For this review, take the finished solid that the model builds, in its own axes (mm). Face numbers are marked on the shaded views. A direction names the side the tool comes from. Round coordinates to 2 decimals unless told otherwise and drop trailing zeros. Order: outer loops, then holes, each group sorted by start corner. A loop starts at its lowest first (then second) coordinate and runs counter-clockwise, first axis right, second up. Notation, with made-up numbers: (-37.5, -34) -> (-21.5, -34) arc R24 cw to (-21.5, 3) -> close; hole circle Ø8 at (-11, 61.25). An arc over 180 degrees is marked (long way). Use a Markdown table: item, result. Add a question column.
1) Consider section C-C (x = 23.5). State the section outline as (y, z) points.
2) Consider section B-B (y = 27). State the section outline as (x, z) points.
3) Consider section A-A (z = 44). State the section outline as (x, y) points, plus the area to 3 significant figures.
4) Consider section D-D (z = 64.5). State the section outline as (x, y) points.
5) Draft analysis for pull direction Z (two halves, no side actions). For the marked faces 1, 2, 3 and 4, state which applies: pulls with the +Z half, pulls with the -Z half, needs draft (parallel to the pull), parting line crosses it, or undercut.
6) Wall thickness on line 1 along Y through (x, z) = (27, 21); line 2 along X through (y, z) = (3.5, 58); line 3 along Y through (x, z) = (91.5, 16): over which ranges is each line inside the solid? List them lowest first. Write a range as [from, to].
7) Clearance check with flat-ended pins moving along their axes: P1, Ø6, axis at x = 12.5, z = 14.5, coming from the +Y side; P2, Ø10, axis at x = 87.5, y = 42, coming from the +Z side; P3, Ø10, axis at y = 23.5, z = 76.5, coming from the +X side; P4, Ø1, axis at x = 19.5, y = 14.5, coming from the +Z side. State where each tip first meets the part, or that it passes through.
8) Machinability: for the marked faces 5, 6 and 7, which of the approach directions +Z, -Z, +X, -X, +Y, -Y give a long, thin tool a straight path to every point of the face, cutting with its end or side? Answer none if there is none.
```python
from build123d import *

# Parameters (mm, degrees)
SKETCH1_W           = 100
SKETCH1_H           = 30
BOSS_EXTRUDE1_DEPTH = 110
SKETCH2_W           = 90
SKETCH2_H           = 10
CUT_EXTRUDE1_DEPTH  = 110
BOSS_EXTRUDE2_DEPTH = 20
CUT_EXTRUDE2_DEPTH  = 20
SKETCH5_W           = 50
SKETCH5_H           = 50
CUT_EXTRUDE3_DEPTH  = 20
CUT_EXTRUDE4_DEPTH  = 20


with BuildPart() as part:
    # Sketch1 → Boss-Extrude1 (new body)
    with BuildSketch(Plane.XY):
        with Locations((50, 15)):
            Rectangle(SKETCH1_W, SKETCH1_H)
    extrude(amount=BOSS_EXTRUDE1_DEPTH)

    # Sketch2 → Cut-Extrude1 (cut)
    with BuildSketch(Plane.ZY):
        with Locations((65, 25)):
            Rectangle(SKETCH2_W, SKETCH2_H)
    extrude(amount=-CUT_EXTRUDE1_DEPTH, mode=Mode.SUBTRACT)

    # Sketch3 → Boss-Extrude2 (add)
    with BuildSketch(Plane.XY.offset(20)):
        with BuildLine():
            Line((20, 30), (80, 30))
            ThreePointArc((80, 30), (50, 60), (20, 30))
        make_face()
    extrude(amount=-BOSS_EXTRUDE2_DEPTH)

    # Sketch4 → Cut-Extrude2 (cut)
    with BuildSketch(Plane(origin=(0, 20, 0), x_dir=(1, 0, 0), z_dir=(0, 1, 0))):
        with BuildLine():
            Line((50, -110), (100, -110))
            Line((100, -110), (100, -60))
            ThreePointArc((100, -60), (85.355339059, -95.355339059), (50, -110))
        make_face()
    extrude(amount=-CUT_EXTRUDE2_DEPTH, mode=Mode.SUBTRACT)

    # Sketch5 → Cut-Extrude3 (cut)
    with BuildSketch(Plane(origin=(0, 20, 0), x_dir=(1, 0, 0), z_dir=(0, 1, 0))):
        with Locations((25, -85)):
            Rectangle(SKETCH5_W, SKETCH5_H)
    extrude(amount=-CUT_EXTRUDE3_DEPTH, mode=Mode.SUBTRACT)

    # Sketch6 → Cut-Extrude4 (cut)
    with BuildSketch(Plane(origin=(0, 20, 0), x_dir=(1, 0, 0), z_dir=(0, 1, 0))):
        with BuildLine():
            Line((20, -60), (50, -60))
            Line((50, -60), (50, -90))
            ThreePointArc((50, -90), (71.213203436, -38.786796564), (20, -60))
        make_face()
    extrude(amount=-CUT_EXTRUDE4_DEPTH, mode=Mode.SUBTRACT)


solid = part.part
```
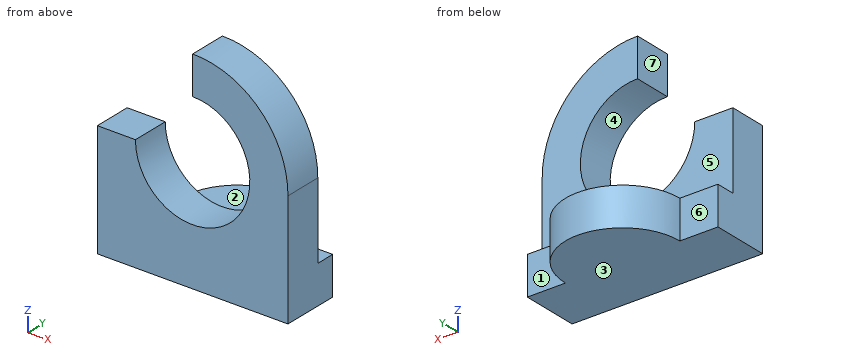
Results list:
| question | item | result |
|---|---|---|
| 1 | outline | (0, 0) -> (44.06, 0) -> (44.06, 20) -> (20, 20) -> (20, 45.94) -> (0, 45.94) -> close |
| 2 | outline | (0, 0) -> (100, 0) -> (100, 20) -> (0, 20) -> close |
| 3 | outline | (0, 0) -> (24.62, 0) -> (24.62, 20) -> (0, 20) -> close; (75.38, 0) -> (100, 0) -> (100, 20) -> (75.38, 20) -> close |
| 3 | area | 985 mm2 |
| 4 | outline | (79.66, 0) -> (99.8, 0) -> (99.8, 20) -> (79.66, 20) -> close |
| 5 | face 1 | needs draft |
| 5 | face 2 | pulls with the +Z half |
| 5 | face 3 | pulls with the -Z half |
| 5 | face 4 | undercut |
| 6 | line 1 | [0, 20] |
| 6 | line 2 | [0, 20.07], [79.93, 100] |
| 6 | line 3 | [0, 30] |
| 7 | P1 | y = 30 |
| 7 | P2 | through |
| 7 | P3 | x = 98.3 |
| 7 | P4 | z = 60 |
| 8 | face 5 | +Z, +X, -X, +Y |
| 8 | face 6 | +Z, -Z, -X, +Y |
| 8 | face 7 | +Z, -X, +Y, -Y |
